Print and shaded views of the part. All mm, measured from the part's lowest x, y and z. Round coordinates to 2 decimals unless told otherwise and drop trailing zeros. Order: outer loops, then holes, each group sorted by start corner. A loop starts at its lowest first (then second) coordinate and runs counter-clockwise, first axis right, second up. Notation, with made-up numbers: (61, 58.25) -> (73, 58.25) arc R9 ccw to (73, 67.25) -> close; hole circle Ø1 at (46.5, 25). An arc over 180 degrees is marked (long way). Answer as CSV lines item,"result". Start each with the question number.
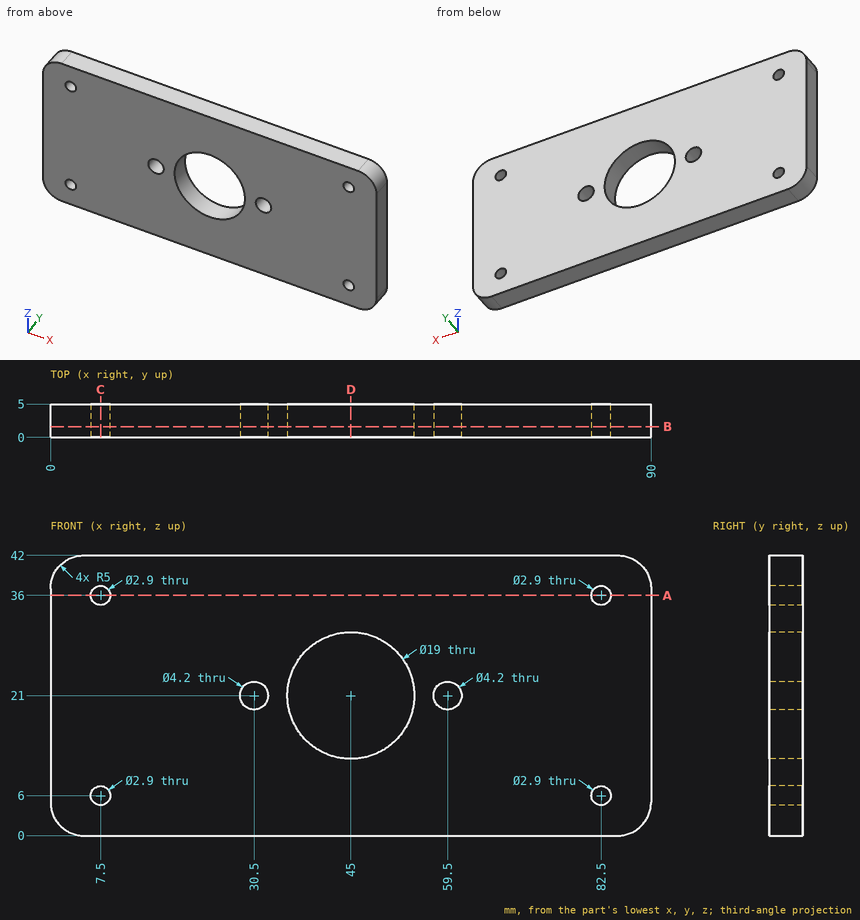
Item 1: Probe line 1 (X direction, y = 3.65, z = 6); line 2 (X direction, y = 1.5, z = 21); line 3 (Z direction, x = 7.5, y = 0.9). List the from-to ranges inside material, lowest first.
Item 2: Band-saw the part on B-B, the plane y = 1.6. Give the cut face in (x, z), and give its area (3 significant figures).
Item 3: Band-saw the part on D-D, the plane x = 45. Give the cut face in (y, z).
Item 4: Band-saw the part on C-C, the plane x = 7.5. Give the cut face in (y, z).
Item 5: Band-saw the part on A-A, the plane z = 36. Give the cut face in (x, y), and give its area (3 significant figures).
Values:
1,line 1,"0 to 6.05, 8.95 to 81.05, 83.95 to 90"
1,line 2,"0 to 28.4, 32.6 to 35.5, 54.5 to 57.4, 61.6 to 90"
1,line 3,"0 to 4.55, 7.45 to 34.55, 37.45 to 42"
2,outline,"(0, 5) arc R5 ccw to (5, 0) -> (85, 0) arc R5 ccw to (90, 5) -> (90, 37) arc R5 ccw to (85, 42) -> (5, 42) arc R5 ccw to (0, 37) -> close; hole circle Ø2.9 at (7.5, 6); hole circle Ø2.9 at (7.5, 36); hole circle Ø4.2 at (30.5, 21); hole circle Ø19 at (45, 21); hole circle Ø4.2 at (59.5, 21); hole circle Ø2.9 at (82.5, 6); hole circle Ø2.9 at (82.5, 36)"
2,area,"3,420 mm²"
3,outline,"(0, 0) -> (5, 0) -> (5, 11.5) -> (0, 11.5) -> close; (0, 30.5) -> (5, 30.5) -> (5, 42) -> (0, 42) -> close"
4,outline,"(0, 0) -> (5, 0) -> (5, 4.55) -> (0, 4.55) -> close; (0, 7.45) -> (5, 7.45) -> (5, 34.55) -> (0, 34.55) -> close; (0, 37.45) -> (5, 37.45) -> (5, 42) -> (0, 42) -> close"
5,outline,"(0, 0) -> (6.05, 0) -> (6.05, 5) -> (0, 5) -> close; (8.95, 0) -> (81.05, 0) -> (81.05, 5) -> (8.95, 5) -> close; (83.95, 0) -> (90, 0) -> (90, 5) -> (83.95, 5) -> close"
5,area,"421 mm²"
